from build123d import *

# Parameters (mm, degrees)
CROQUIS2_W              = 450
CROQUIS2_H              = 300
SALIENTE_EXTRUIR1_DEPTH = 100
CROQUIS4_W              = 100
CROQUIS4_H              = 15
SALIENTE_EXTRUIR2_DEPTH = 9
CROQUIS5_W              = 100
CROQUIS5_H              = 15
SALIENTE_EXTRUIR3_DEPTH = 9


with BuildPart() as part:
    # Croquis2 → Saliente-Extruir1 (new body)
    with BuildSketch(Plane(origin=(0, 0, 0), x_dir=(0, 0, -1), z_dir=(1, 0, 0))):
        Rectangle(CROQUIS2_W, CROQUIS2_H)
    extrude(amount=SALIENTE_EXTRUIR1_DEPTH)

    # Croquis4 → Saliente-Extruir2 (add)
    with BuildSketch(Plane(origin=(0, 0, -225), x_dir=(-1, 0, 0), z_dir=(0, 0, -1))):
        with Locations((-50, 142.5)):
            Rectangle(CROQUIS4_W, CROQUIS4_H)
    extrude(amount=SALIENTE_EXTRUIR2_DEPTH)

    # Croquis5 → Saliente-Extruir3 (add)
    with BuildSketch(Plane.XY.offset(225)):
        with Locations((50, 142.5)):
            Rectangle(CROQUIS5_W, CROQUIS5_H)
    extrude(amount=SALIENTE_EXTRUIR3_DEPTH)


solid = part.part
Work out the finished part from the listing and answer in its coordinate system (mm). A direction names the side the tool comes from. Give positions to 0.01 mm unless a question says otherwise; leave off trailing zeros. Loops run counter-clockwise (first coordinate to the right, second up) from the corner with the lowest first, then second, coordinate; pieces in that order, holes last. Notation, with made-up numbers: (-10.75, -34) - (31.25, -34) arc R25 ccw to (31.25, -14) - close; hole circle Ø5 at (-34, 5.5). An arc over 180 degrees is marked (long way). Answer in a Markdown table with one row per item. Add a question column.
Q1. Each of these flat-tipped pins is pushed along its axis until it touches: P1, Ø5, axis at x = 10, y = 78, coming from the +Z side; P2, Ø7, axis at x = 48.5, z = -230.5, coming from the -Y side; P3, Ø3, axis at x = 22, y = -36, coming from the -Z side; P4, Ø10, axis at y = 39.5, z = 128.5, coming from the -X side. Where does it stop, or does it pass through?
Q2. The part is cut by section B-B (y = -114.5). Determine the outline of the cut face in (x, z).
Q3. The part is cut by section A-A (x = 33). Determine the outline of the cut face in (y, z).
Q4. Consider line 1 along Z through (x, y) = (21, 53). Determine where the line is inside the solid, lowest interval first.
Q5. A tool of negligible diameter and unlimited length cuts with its end or side. For faces 1 (the flat face through (49, -9, -225)), 2 (the flat face through (49, 135, 229)), 3 (the flat face through (100, -2, -3)), from which of +Z, -Z, +X, -X, +Y, -Y can it reach the whole face along a straight path? Write none if from no direction.
Solution:
| question | item | result |
|---|---|---|
| 1 | P1 | stops at z = 225 |
| 1 | P2 | stops at y = 135 |
| 1 | P3 | stops at z = -225 |
| 1 | P4 | stops at x = 0 |
| 2 | outline | (0, -225) - (100, -225) - (100, 225) - (0, 225) - close |
| 3 | outline | (-150, -225) - (135, -225) - (135, -234) - (150, -234) - (150, 234) - (135, 234) - (135, 225) - (-150, 225) - close |
| 4 | line 1 | z = -225 to 225 |
| 5 | face 1 | -Z, +X, -X, -Y |
| 5 | face 2 | +Z, +X, -X, -Y |
| 5 | face 3 | +Z, -Z, +X, +Y, -Y |
